Autodesk Inventor part; units mm, degrees
ref_plane "YZ Plane" through (0, 0, 0) normal (1, 0, 0) x (0, 1, 0)
ref_plane "XZ Plane" through (0, 0, 0) normal (0, 1, 0) x (-1, 0, 0)
ref_plane "XY Plane" through (0, 0, 0) normal (0, 0, 1) x (1, 0, 0)
sketch "スケッチ1" plane through (0, 0, 0) normal (0, 0, 1) x (1, 0, 0)
  line L0 (55, -93.4) -> (-55, -93.4)
  line L1 (-55, -93.4) -> (-55, 75)
  line L2 (-55, 75) -> (55, 75)
  line L3 (55, 75) -> (55, -93.4)
  line L4 (55, -93.4) -> (-55, 75) construction
  line L5 (-55, -93.4) -> (55, 75) construction
  point P0 (0, 0)
  point P1 (0, -9.2)
  point P2 (0, -9.2)
  dimension "d50" = 93.4
  dimension "d51" = 110
  dimension "d52" = 75
extrude "プレート1" add sketch "スケッチ1" along normal blind 2
sketch "スケッチ3" plane through (0, 0, 2) normal (0, 0, 1) x (1, 0, 0)
  circle A0 centre (0, 38.4) radius 19
  circle A1 centre (0, -38.4) radius 10
  point P0 (0, 0)
  dimension "d22" = 38
  dimension "d53" = 20
  dimension "d55" = 76.8
  dimension "d56" = 38.4
extrude "押し出し1" cut sketch "スケッチ3" against normal blind 10 contours A0
sketch "スケッチ2" plane through (0, 0, 2) normal (0, 0, 1) x (1, 0, 0)
  circle A0 centre (0, 38.4) radius 15 construction
  circle A1 centre (0, -38.4) radius 53.5
  point P0 (0, 0)
  point P1 (0, 53.4)
  point P2 (-15, 38.4)
  point P3 (0, 23.4)
  point P4 (15, 38.4)
  point P5 (-46.3324, -11.65)
  point P6 (-53.5, -38.4)
  point P7 (-46.3324, -65.15)
  point P8 (-26.75, -84.7324)
  point P9 (0, -91.9)
  point P10 (26.75, -84.7324)
  point P11 (46.3324, -65.15)
  point P12 (53.5, -38.4)
  point P13 (46.3324, -11.65)
  point P14 (26.75, 7.9324)
  point P15 (0, 15.1)
  point P16 (-26.75, 7.9324)
  dimension "d3" = 30
  dimension "d8" = 107
  dimension "d6" = 360
  dimension "d11" = 360
  dimension "d13" = 76.8
  dimension "d14" = 38.4
  dimension "d58" = 0
hole "穴1" at (-26.75, -84.7324, 2) at (-46.3324, -65.15, 2) at (-26.75, 7.9324, 2) at (-46.3324, -11.65, 2) at (26.75, 7.9324, 2) at (46.3324, -11.65, 2) at (46.3324, -65.15, 2) at (26.75, -84.7324, 2) direction (0, 0, -1) diameter 3.2 end through all
sketch "スケッチ4" plane through (0, 0, 2) normal (0, 0, 1) x (1, 0, 0)
  line L0 (55, -93.4) -> (-55, -93.4)
  line L1 (-55, -93.4) -> (-55, 75)
  line L2 (55, 75) -> (55, -93.4)
  line L3 (-55, 75) -> (55, 75)
  line L4 (-50, 70) -> (-50, -88.4)
  line L5 (-50, -88.4) -> (50, -88.4)
  line L6 (50, -88.4) -> (50, 70)
  line L7 (50, 70) -> (-50, 70)
  point P0 (-50, 0)
  point P1 (50, 0)
  point P2 (0, 0)
  dimension "d57" = 5
hole "穴2" at (-50, -88.4, 2) at (50, -88.4, 2) at (50, 70, 2) at (-50, 70, 2) at (-50, 0, 2) at (50, 0, 2) direction (0, 0, -1) diameter 4.3 end through all
fillet "コーナーR1" radius 5 4 edges at (-55, -93.4, 1) (55, -93.4, 1) (55, 75, 1) (-55, 75, 1)
sketch "スケッチ5" plane through (0, 0, 2) normal (0, 0, 1) x (1, 0, 0)
  circle A0 centre (0, -38.4) radius 41
  point P0 (0, 0)
  dimension "d35" = 82
extrude "押し出し2" cut sketch "スケッチ5" against normal blind 10
sketch "スケッチ6" plane through (0, 0, 2) normal (0, 0, 1) x (1, 0, 0)
  circle A0 centre (0, 38.4) radius 19
  circle A1 centre (0, 38.4) radius 27
  point P0 (0, 0)
  point P1 (-23.3827, 51.9)
  point P2 (-23.3827, 24.9)
  point P3 (0, 11.4)
  point P4 (23.3827, 24.9)
  point P5 (23.3827, 51.9)
  point P6 (0, 65.4)
  dimension "d38" = 54
  dimension "d41" = 360
  dimension "d59" = 0
hole "穴3" at (0, 65.4, 2) at (23.3827, 51.9, 2) at (23.3827, 24.9, 2) at (-23.3827, 24.9, 2) at (-23.3827, 51.9, 2) direction (0, 0, -1) diameter 4.3 end through all
sketch "スケッチ7" plane through (0, 0, 2) normal (0, 0, 1) x (1, 0, 0)
  circle A0 centre (-50, 0) radius 2.15
  line L0 (-46.2, 0) -> (-50, 0) construction
  line L1 (-46.2, 2.15) -> (-50, 2.15)
  line L2 (-50, -2.15) -> (-46.2, -2.15)
  arc A1 (-46.2, -2.15) -> (-46.2, 2.15) centre (-46.2, 0) ccw
  arc A2 (-50, 2.15) -> (-50, -2.15) centre (-50, 0) ccw
  point P0 (0, 0)
  point P1 (-48.1, 0)
  dimension "d60" = 48.1
extrude "押し出し3" cut sketch "スケッチ7" against normal through all
equation "\"d20\" = Thickness"
equation "\"d2\" = Thickness"
equation "\"BendRadius\" = Thickness"
equation "\"BendReliefWidth\" = Thickness"
equation "\"BendReliefDepth\" = 0.5 * Thickness"
equation "\"CornerReliefSize\" = 4 * Thickness"
equation "\"MinimumRemnant\" = 2 * Thickness"
equation "\"TransitionRadius\" = BendRadius"
equation "\"JacobiRadiusSize\" = BendRadius"
equation "\"GapSize\" = Thickness"
properties part number "carbonplate3" material "CFRP"
Part model, mm, in its own coordinate system. Round coordinates to 2 decimals unless told otherwise and drop trailing zeros. Write each loop counter-clockwise with the first axis right and the second up, starting at its lowest first coordinate (ties: lowest second). Pieces come first, ordered by that corner, then holes. Notation, with made-up numbers: M 49.5,-3 L 104.5,-3 A24 ccw 104.5,27 Z; hole C 32,43 d6. An arc over 180 degrees is marked long. Return JSON: item names as keys, results as strings. Group by question number.
(1) Two-plate mould, pull along Y, no slides. Class faces 1 (the face through (-47.68, -12.51, 0.99)), 2 (the face through (-53.57, -91.9, 1.01)), 3 (the face through (-1, 11, 0)): +Y half, -Y half, draft (parallel to the pull), parting line (faces both ways), or undercut.
(2) Saw through at D-D on y = 65.4. Write the cut outline in (x, z).
(3) Drill centre lines: probe 1 along Y at (x, z) = (50, 0.5); probe 2 along X at (y, z) = (51.9, 0.6). Where is each one in solid material? Low to high.
(4) Pin check, flat tip, straight feed: pin 1 Ø2.5 at (x, y) = (23.38, 51.9) entering from +Z. Stop position of the tip, or through.
(5) Saw through at B-B on x = 0. Write the cut outline in (y, z).
(6) Saw through at A-A on y = -53.5. Write the cut outline in (x, z).
(7) Saw through at C-C on z = 0.7. Count the separate pieces of the cut face and the enclosed holes in it, then the cut area to 3 significant figures.
Returned:
{
 "1": {"face 1": "undercut", "face 2": "-Y half", "face 3": "draft"},
 "2": {"outline": "M -55,0 L -2.15,0 L -2.15,2 L -55,2 Z; M 2.15,0 L 55,0 L 55,2 L 2.15,2 Z"},
 "3": {"probe 1": "-93.4 to -90.55, -86.25 to -2.15, 2.15 to 67.85, 72.15 to 75", "probe 2": "-55 to -25.53, -21.23 to -13.37, 13.37 to 21.23, 25.53 to 55"},
 "4": {"pin 1": "through"},
 "5": {"outline": "M -93.4,0 L -79.4,0 L -79.4,2 L -93.4,2 Z; M 2.6,0 L 19.4,0 L 19.4,2 L 2.6,2 Z; M 57.4,0 L 63.25,0 L 63.25,2 L 57.4,2 Z; M 67.55,0 L 75,0 L 75,2 L 67.55,2 Z"},
 "6": {"outline": "M -55,0 L -38.12,0 L -38.12,2 L -55,2 Z; M 38.12,0 L 55,0 L 55,2 L 38.12,2 Z"},
 "7": {"separate pieces": "1", "enclosed holes": "21", "area": "11,800 mm²"}
}
